Here's the drawing with two shaded views (mm, measured from the low corner). I have some questions. A direction names the side the tool comes from. Round coordinates to 2 decimals unless told otherwise and drop trailing zeros. Loops run counter-clockwise (first coordinate to the right, second up) from the corner with the lowest first, then second, coordinate; pieces in that order, holes last. Notation, with made-up numbers: M 71,62.25 L 84,62.25 A26 ccw 84,79.25 Z; hole C 45,18.25 d6. An arc over 180 degrees is marked long. Answer as CSV lines item,"result".
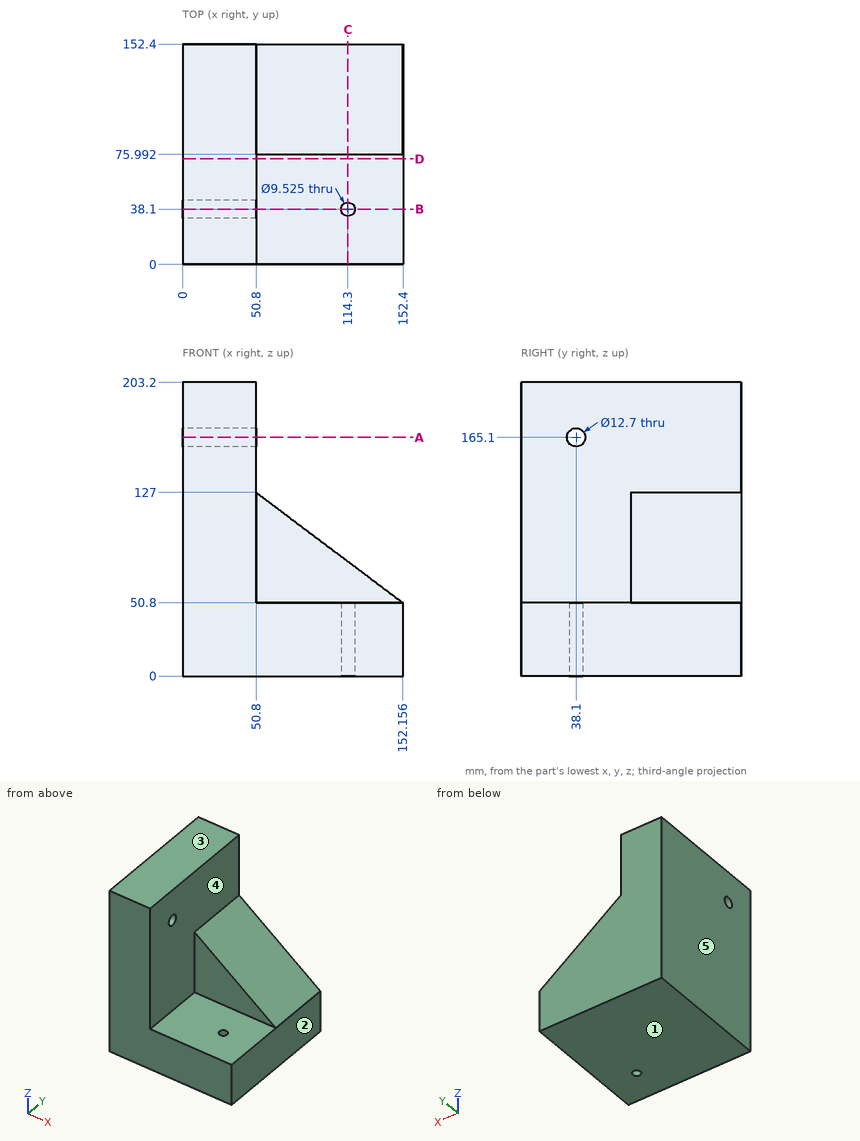
1. I want a section at D-D, the plane y = 73. Please give me the cut outline in (x, z), and give its area (3 significant figures).
Evaluation:
outline,"M 0,0 L 152.4,0 L 152.4,50.8 L 50.8,50.8 L 50.8,203.2 L 0,203.2 Z"
area,"15,500 mm²"
2. I want a section at C-C, the plane x = 114.3. Please give me the cut outline in (y, z).
Evaluation:
outline,"M 0,0 L 33.34,0 L 33.34,50.8 L 0,50.8 Z; M 42.86,0 L 152.4,0 L 152.4,79.26 L 75.99,79.26 L 75.99,50.8 L 42.86,50.8 Z"
3. I want a section at B-B, the plane y = 38.1. Please give me the cut outline in (x, z), and give its area (3 significant figures).
Evaluation:
outline,"M 0,0 L 109.54,0 L 109.54,50.8 L 50.8,50.8 L 50.8,158.75 L 0,158.75 Z; M 0,171.45 L 50.8,171.45 L 50.8,203.2 L 0,203.2 Z; M 119.06,0 L 152.4,0 L 152.4,50.8 L 119.06,50.8 Z"
area,"14,400 mm²"
4. For P1, Ø1, axis at x = 86, y = 61.5, coming from the +Z side, with a flat end and sliding along its axis, tell me the tip position at first contact or that it passes through.
Evaluation:
P1,"stops at z = 50.8"
5. If I drill on line 1 (X direction, y = 38, z = 29); line 2 (Z direction, x = 31, y = 38); line 3 (Y direction, x = 25, z = 165), over which ranges is the centre line in solid material (lowest first)? Write a range as [from, to].
Evaluation:
line 1,"x = [0, 109.54], [119.06, 152.4]"
line 2,"z = [0, 158.75], [171.45, 203.2]"
line 3,"y = [0, 31.75], [44.45, 152.4]"
6. I want a section at A-A, the plane z = 165.1. Please give me the cut outline in (x, y).
Evaluation:
outline,"M 0,0 L 50.8,0 L 50.8,31.75 L 0,31.75 Z; M 0,44.45 L 50.8,44.45 L 50.8,152.4 L 0,152.4 Z"
7. Which directions (+Z, -Z, +X, -X, +Y, -Y) give clear straight access to the entire face, cutting with the end or side of a thin tool? Please do the marked faces 4 and 5.
Evaluation:
face 4,"+Z, +X, -Y"
face 5,"+Z, -Z, -X, +Y, -Y"
8. We'd pull the mould along Z, two halves only. Please class the marked faces 1, 2 and 3: pulls with the +Z half, pulls with the -Z half, needs draft (parallel to the pull), parting line crosses it, or undercut.
Evaluation:
face 1,"pulls with the -Z half"
face 2,"needs draft"
face 3,"pulls with the +Z half"
